```python
from build123d import *

# Parameters (mm, degrees)
SKETCH219_W     = 50
SKETCH219_H     = 50
PAD112_DEPTH    = 10
SKETCH220_W     = 30
SKETCH220_H     = 7
POCKET049_DEPTH = 60.001
SKETCH221_R     = 2.1
POCKET050_DEPTH = 10.001
PAD113_DEPTH    = 3
SKETCH223_R     = 2.1
POCKET051_DEPTH = 7
SKETCH224_W     = 15
SKETCH224_H     = 12
POCKET052_DEPTH = 3.001
FILLET070_R     = 3
CHAMFER076_SIZE = 1
FILLET071_R     = 3
CHAMFER077_SIZE = 0.4
CHAMFER078_SIZE = 0.4


with BuildPart() as part:
    # Sketch219 → Pad112 (new body)
    with BuildSketch(Plane.XY):
        with Locations((0, 35)):
            Rectangle(SKETCH219_W, SKETCH219_H)
    extrude(amount=-PAD112_DEPTH)

    # Sketch220 → Pocket049 (cut, through all)
    with BuildSketch(Plane.XZ):
        with Locations((0, -3.5)):
            Rectangle(SKETCH220_W, SKETCH220_H)
    extrude(amount=-POCKET049_DEPTH, mode=Mode.SUBTRACT)

    # Sketch221 → Pocket050 (cut, through all)
    with BuildSketch(Plane.XY):
        with Locations((-20, 35)):
            Circle(SKETCH221_R)
        with Locations((20, 35)):
            Circle(SKETCH221_R)
    extrude(amount=-POCKET050_DEPTH, mode=Mode.SUBTRACT)

    # Sketch222 (on Face8 of Pocket050) → Pad113 (join)
    with BuildSketch(Plane.XY.offset(-7)):
        with BuildLine():
            ThreePointArc((5, 45), (0, 50), (-5, 45))
            Line((-5, 45), (-5, 32))
            ThreePointArc((-5, 32), (0, 27), (5, 32))
            Line((5, 32), (5, 45))
        make_face()
    extrude(amount=PAD113_DEPTH)

    # Sketch223 (on Face17 of Pad113) → Pocket051 (cut)
    with BuildSketch(Plane.XY.offset(-4)):
        with Locations((0, 45)):
            Circle(SKETCH223_R)
        with Locations((0, 32)):
            Circle(SKETCH223_R)
    extrude(amount=-POCKET051_DEPTH, mode=Mode.SUBTRACT)

    # Sketch224 (on Face8 of Pocket051) → Pocket052 (cut, through all)
    with BuildSketch(Plane.XY.offset(-7)):
        with Locations((0, 16)):
            Rectangle(SKETCH224_W, SKETCH224_H)
    extrude(amount=-POCKET052_DEPTH, mode=Mode.SUBTRACT)

    # Fillet070
    fillet070_edges = [part.edges().sort_by_distance(p)[0] for p in [
        (-7.5, 10, -8.5),
        (7.5, 10, -8.5),
        (-7.5, 22, -8.5),
        (7.5, 22, -8.5),
    ]]
    fillet(fillet070_edges, radius=FILLET070_R)

    # Chamfer076
    chamfer076_edges = [part.edges().sort_by_distance(p)[0] for p in [
        (-22.1, 35, 0),
        (-22.1, 35, -10),
        (-2.1, 32, -4),
        (-2.1, 32, -10),
        (-2.1, 45, -4),
        (-2.1, 45, -10),
        (17.9, 35, 0),
        (17.9, 35, -10),
    ]]
    chamfer(chamfer076_edges, length=CHAMFER076_SIZE)

    # Fillet071
    fillet071_edges = [part.edges().sort_by_distance(p)[0] for p in [
        (-25, 10, -5),
        (-25, 60, -5),
        (25, 60, -5),
        (25, 10, -5),
        (-15, 10, -3.5),
        (-15, 60, -3.5),
        (15, 60, -3.5),
        (15, 10, -3.5),
    ]]
    fillet(fillet071_edges, radius=FILLET071_R)

    # Chamfer077
    chamfer077_edges = [part.edges().sort_by_distance(p)[0] for p in [
        (8.37868, 10.87868, -10),
    ]]
    chamfer(chamfer077_edges, length=CHAMFER077_SIZE)

    # Chamfer078
    chamfer078_edges = [part.edges().sort_by_distance(p)[0] for p in [
        (-20, 10, 0),
        (20, 10, 0),
        (0, 27, -4),
        (0, 27, -7),
        (-12.75, 10, -7),
        (0, 60, -7),
    ]]
    chamfer(chamfer078_edges, length=CHAMFER078_SIZE)


with BuildPart() as part_1:
    # Body097 placement: moved
    add(part.part.moved(Location((0, 0, 320))))


solid = part_1.part
```
Read the model definition and answer for the solid it produces. Units are mm, in the model's axes. A direction names the side the tool comes from. Coordinates: 2 decimals unless noted, no trailing zeros. Loops run counter-clockwise (first coordinate to the right, second up) from the corner with the lowest first, then second, coordinate; pieces in that order, holes last.
(1) The part is cut by section A-A (x = 0). Count the separate pieces of the cut face and the enclosed holes in it, and give its area (3 significant figures).
Solution:
separate pieces: 3
enclosed holes: 0
area: 128 mm2
(2) The part is cut by section C-C (x = 20). Determine the outline of the cut face in (y, z).
Solution:
outline: (10, 310.4) - (10.4, 310) - (31.9, 310) - (32.9, 311) - (32.9, 319) - (31.9, 320) - (10.4, 320) - (10, 319.6) - close; (37.1, 311) - (38.1, 310) - (59.6, 310) - (60, 310.4) - (60, 319.6) - (59.6, 320) - (38.1, 320) - (37.1, 319) - close
(3) A tool of negligible diameter and unlimited length cuts with its end or side. For faces 5 (the face through (6.64, 21.1, 311.48)), 6 (the face through (8.61, 11.06, 312.89)), 7 (the face through (16.11, 58.94, 319.89)), 8 (the face through (15, 35, 316)), from which of +Z, -Z, +X, -X, +Y, -Y can it reach the whole face along a straight path? Write none if from no direction.
Solution:
face 5: +Z, -Z, -Y
face 6: +Z, -Y
face 7: +Z, +Y
face 8: +Z, +Y, -Y
(4) The mould has two halves that part along X. Classify faces 1 (the face through (0.1, 49.71, 315.89)), 2 (the face through (23.94, 11.102, 310.114)), 3 (the face through (-15, 35, 316)), 4 (the face through (16, 35, 320)): released by +X, released by -X, zero draft, split by the parting line, or undercut.
Solution:
face 1: undercut
face 2: released by +X
face 3: undercut
face 4: zero draft
(5) The part is cut by section B-B (z = 317.25). Determine the outline of the cut face in (x, y), and give its area (3 significant figures).
Solution:
outline: (-25, 13) arc R3 ccw to (-22, 10) - (-18, 10) arc R3 ccw to (-15, 13) - (-15, 57) arc R3 ccw to (-18, 60) - (-22, 60) arc R3 ccw to (-25, 57) - close; (15, 13) arc R3 ccw to (18, 10) - (22, 10) arc R3 ccw to (25, 13) - (25, 57) arc R3 ccw to (22, 60) - (18, 60) arc R3 ccw to (15, 57) - close; hole circle Ø4.2 at (-20, 35); hole circle Ø4.2 at (20, 35)
area: 957 mm2
(6) The part is cut by section D-D (y = 16.5). Determine the outline of the cut face in (x, z).
Solution:
outline: (-25, 310.4) - (-24.6, 310) - (-7.9, 310) - (-7.5, 310.4) - (-7.5, 312.6) - (-7.9, 313) - (-15, 313) - (-15, 319.6) - (-15.4, 320) - (-24.6, 320) - (-25, 319.6) - close; (7.5, 310.4) - (7.9, 310) - (24.6, 310) - (25, 310.4) - (25, 319.6) - (24.6, 320) - (15.4, 320) - (15, 319.6) - (15, 313) - (7.9, 313) - (7.5, 312.6) - close
(7) Consider line 1 along X through (y, z) = (42, 315.5); line 2 along Y through (x, z) = (0, 312.2); line 3 along X through (y, z) = (20, 317.5). Determine where each line is inside the solid, lowest interval first.
Solution:
line 1: x = -25 to -15, -5 to 5, 15 to 25
line 2: y = 22 to 29.9, 34.1 to 42.9, 47.1 to 60
line 3: x = -25 to -15, 15 to 25
(8) Flat-ended cylindrical pins translate along their axes: pin 1 Ø5.5 at (x, y) = (-20, 35) entering from -Z; pin 2 Ø2.5 at (x, y) = (0, 32) entering from -Z; pin 3 Ø3 at (x, z) = (-14.5, 317.5) entering from -Y; pin 4 Ø6 at (x, y) = (-4, 54.5) entering from +Z. Find the tip coordinate at first contact, or state that the pin passes through.
Solution:
pin 1: stops at z = 310.35
pin 2: passes through
pin 3: stops at y = 10.76
pin 4: stops at z = 313
